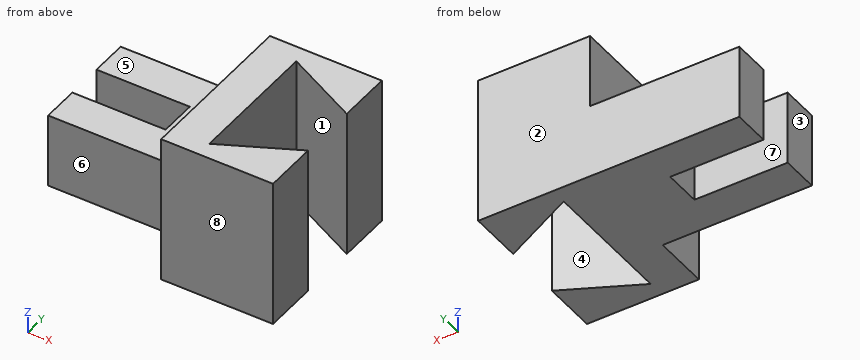
from build123d import *

# Parameters (mm, degrees)
AUFSATZ_LINEAR_AUSTRAGEN1_DEPTH      = 20
SKIZZE2_W                            = 40
SKIZZE2_H                            = 45
AUFSATZ_LINEAR_AUSTRAGEN3_DEPTH      = 30
SCHNITT_LINEAR_AUSTRAGEN1_DEPTH      = 87.02325267
SCHNITT_LINEAR_AUSTRAGEN1_DEPTH_BACK = 40


with BuildPart() as part:
    # Skizze1 → Aufsatz-Linear austragen1 (new body)
    with BuildSketch(Plane.XY):
        Polygon((0, 0), (40, 0), (40, 30), (0, 30), (0, 20), (25, 20), (25, 10), (0, 10), align=None)
    extrude(amount=AUFSATZ_LINEAR_AUSTRAGEN1_DEPTH)

    # Skizze2 → Aufsatz-Linear austragen3 (add)
    with BuildSketch(Plane(origin=(40, 0, 0), x_dir=(0, 0, -1), z_dir=(1, 0, 0))):
        with Locations((-20, 7.5)):
            Rectangle(SKIZZE2_W, SKIZZE2_H)
    extrude(amount=AUFSATZ_LINEAR_AUSTRAGEN3_DEPTH)

    # Skizze3 → Schnitt-Linear austragen1 (cut, two sides: drawn at the far end of the back side and taken through both)
    with BuildSketch(Plane.XY.offset(40).offset(-SCHNITT_LINEAR_AUSTRAGEN1_DEPTH_BACK)):
        Polygon((215.534169047, -57.267084524), (70, 15.5), (50, 25.5), (50, -10.5), (70, -0.5), (215.534169047, 72.267084524), (-109.890125992, 72.267084524), (-109.890125992, -57.267084524), align=None)
    extrude(amount=SCHNITT_LINEAR_AUSTRAGEN1_DEPTH + SCHNITT_LINEAR_AUSTRAGEN1_DEPTH_BACK, mode=Mode.SUBTRACT)


solid = part.part
Input: part model. Units: mm. Frame: model coordinates. Face numbers are marked on the shaded views. A direction names the side the tool comes from. Coordinates: 2 decimals unless noted, no trailing zeros. Write each loop counter-clockwise with the first axis right and the second up, starting at its lowest first coordinate (ties: lowest second). Pieces come first, ordered by that corner, then holes. Notation, with made-up numbers: M 22.25,65 L 64.25,65 A15 cw 64.25,86 Z; hole C -29,0 d11. An arc over 180 degrees is marked long. Answer as a JSON object with one key per item and string values. Group by question number.
(1) Section B-B on y = 16.5. Output: boundary loops of the cut face in (x, z).
(2) Contact query for flat-ended pins moving along their axis: P1, Ø22, axis at x = 19.5, z = 8, coming from the -Y side; P2, Ø5, axis at y = 13.5, z = 11, coming from the -X side; P3, Ø1.5, axis at y = 14.5, z = 24.5, coming from the -X side. Output: stop coordinate, or through.
(3) Set-up query: the marked faces 4, 5, 6, 7 and 8. Return all of +Z, -Z, +X, -X, +Y, -Y with unobstructed straight access to the full face (end or side cutting, diameter ignored); none if empty.
(4) Section C-C on y = -4. Output: boundary loops of the cut face in (x, z), plus the area to 3 significant figures.
(5) Mould query, pull axis X, two halves, no side actions, for the marked faces 1, 2 and 3. Classes: pulls with the +X half, pulls with the -X half, needs draft (parallel to the pull), parting line crosses it, or undercut.
(6) Section A-A on x = 63.5. Output: boundary loops of the cut face in (y, z).
(7) Section D-D on z = 23. Output: boundary loops of the cut face in (x, y), plus the area to 3 significant figures.
(8) Ray query, line 1 along Y through (x, z) = (18.5, 12.5); line 2 along X through (y, z) = (-13, 7.5); line 3 along X through (y, z) = (-6, 29). Return the intervals inside material, ascending. Write a range as [from, to].
Result set:
{
 "1": {"outline": "M 25,0 L 50,0 L 50,40 L 40,40 L 40,20 L 25,20 Z; M 68,0 L 70,0 L 70,40 L 68,40 Z"},
 "2": {"P1": "stops at y = 0", "P2": "stops at x = 25", "P3": "stops at x = 40"},
 "3": {"face 4": "+Z, -Z", "face 5": "+Z, -X, +Y, -Y", "face 6": "+Z, -Z, -X, -Y", "face 7": "+Z, -Z, -X", "face 8": "+Z, -Z, +X, -X, -Y"},
 "4": {"outline": "M 40,0 L 50,0 L 50,40 L 40,40 Z; M 63,0 L 70,0 L 70,40 L 63,40 Z", "area": "680 mm2"},
 "5": {"face 1": "undercut", "face 2": "needs draft", "face 3": "pulls with the -X half"},
 "6": {"outline": "M -15,0 L -3.75,0 L -3.75,40 L -15,40 Z; M 18.75,0 L 30,0 L 30,40 L 18.75,40 Z"},
 "7": {"outline": "M 40,-15 L 70,-15 L 70,-0.5 L 50,-10.5 L 50,25.5 L 70,15.5 L 70,30 L 40,30 Z", "area": "830 mm2"},
 "8": {"line 1": "y = [0, 10], [20, 30]", "line 2": "x = [40, 70]", "line 3": "x = [40, 50], [59, 70]"}
}
